Design review of the part built by this model. Coordinates are the model's own, in mm. Face numbers are marked on the shaded views. A direction names the side the tool comes from. Round coordinates to 2 decimals unless told otherwise and drop trailing zeros. Loops run counter-clockwise (first coordinate to the right, second up) from the corner with the lowest first, then second, coordinate; pieces in that order, holes last. Notation, with made-up numbers: (56.5, 40) - (73.5, 40) arc R21 cw to (73.5, 54) - close; hole circle Ø5 at (-25, 74). An arc over 180 degrees is marked (long way). Use one line per item in the form item = value. Start each with the question number.
(1) We need section C-C, the plane z = 3. Write out the cut boundary in (x, y).
(2) We need section D-D, the plane z = 16. Write out the cut boundary in (x, y).
(3) The part is to be moulded in two halves that separate along X. For the marked faces 6, 7, 8 and 9, say which applies: released by +X, released by -X, zero draft, split by the parting line, or undercut.
(4) We need section A-A, the plane y = -40. Write out the cut boundary in (x, z), then the cut area to 3 significant figures.
(5) For pin 1 (5 mm diameter, centred on x = -23.5, y = -33, fed in from -Z); pin 2 (4 mm diameter, centred on x = 20.5, y = -42.5, fed in from +Z); pin 3 (9.5 mm diameter, centred on x = -24, y = -44, fed in from +Z), all flat-tipped, find the tip position at first contact; note any pin that passes through.
(6) Machinability: for the marked faces 1, 2, 3, 4 and 5, which of the approach directions +Z, -Z, +X, -X, +Y, -Y give a long, thin tool a straight path to every point of the face, cutting with its end or side? Answer none if there is none.
(7) Wall thickness on probe 1 along Y at (x, z) = (1.5, 14); probe 2 along Y at (x, z) = (4, 12.25); probe 3 along Z at (x, y) = (-19, -17.5): over which ranges is each line inside the solid? List them lowest first. Write a range as [from, to].
(8) We need section B-B, the plane x = -8.5. Write out the cut boundary in (y, z), then the cut area to 3 significant figures.
from build123d import *

# Parameters (mm, degrees)
F0_W      = 100
F0_H      = 60
F1_DEPTH  = 31
F3_DEPTH  = 60.001
F4_W      = 30.1
F4_H      = 44.45
F5_DEPTH  = 26.0514508643
F6_W      = 3.4385170311
F6_H      = 44.45
F7_DEPTH  = 8.2
F8_DEPTH  = 2.2
F9_DEPTH  = 22
F10_W     = 3.7688823059
F10_H     = 44.2940850452
F11_DEPTH = 3.6
F12_W     = 35.5
F12_H     = 4.5
F13_DEPTH = 3.7
F14_DEPTH = 0.8
F15_W     = 12
F15_H     = 44.45
F17_DEPTH = 0.7
F18_W     = 10
F18_H     = 44.45
F19_DEPTH = 0.7
F21_DEPTH = 70.6


with BuildPart() as f1:
    # F0 (on Top) → F1 (new body)
    with BuildSketch(Plane.XY):
        with Locations((0.4987093992, -30)):
            Rectangle(F0_W, F0_H)
    extrude(amount=F1_DEPTH)

    # F2 (on face) → F3 (cut, through all)
    with BuildSketch(Plane.XZ.offset(60)):
        Polygon((-49.5012906008, 26.9820707818), (50.4987093992, 0), (50.4987093992, 31), (-49.5012906008, 31), align=None)
    extrude(amount=-F3_DEPTH, mode=Mode.SUBTRACT)

    # F4 (on face) → F5 (cut, through all)
    with BuildSketch(Plane(origin=(3.4269736671, 0, 12.7009290534), x_dir=(0.9654726309, 0, -0.2605045086), z_dir=(0.2605045086, 0, 0.9654726309))):
        with Locations((-1.0446142405, -30.225)):
            Rectangle(F4_W, F4_H)
    extrude(amount=-F5_DEPTH, mode=Mode.SUBTRACT)

    # F6 (on face) → F7 (cut)
    with BuildSketch(Plane(origin=(3.4269736671, 0, 12.7009290534), x_dir=(0.9654726309, 0, -0.2605045086), z_dir=(0.2605045086, 0, 0.9654726309))):
        with Locations((-17.8138727561, -30.225)):
            Rectangle(F6_W, F6_H)
    extrude(amount=-F7_DEPTH, mode=Mode.SUBTRACT)

    # F8 (add): a face of the model
    f8_faces = [f1.faces().sort_by_distance(p)[0] for p in [
        (15.7275193268, -30.225, 4.5262314589),
    ]]
    extrude(f8_faces, amount=F8_DEPTH)

    # F9 (cut): a face of the model
    f9_faces = [f1.faces().sort_by_distance(p)[0] for p in [
        (-49.5012906008, -30, 13.4910353909),
    ]]
    extrude(f9_faces, amount=-F9_DEPTH, mode=Mode.SUBTRACT)

    # F10 (on face) → F11 (join)
    with BuildSketch(Plane(origin=(3.4269736671, 0, 12.7009290534), x_dir=(0.9654726309, 0, -0.2605045086), z_dir=(0.2605045086, 0, 0.9654726309))):
        with Locations((13.6898269124, -30.3029574774)):
            Rectangle(F10_W, F10_H)
    extrude(amount=F11_DEPTH)

    # F12 (on face) → F13 (join)
    with BuildSketch(Plane(origin=(3.4269736671, 0, 12.7009290534), x_dir=(0.9654726309, 0, -0.2605045086), z_dir=(0.2605045086, 0, 0.9654726309))):
        with Locations((-1.7831312716, -2.25)):
            Rectangle(F12_W, F12_H)
        with Locations((-1.7831312716, -57.75)):
            Rectangle(F12_W, F12_H)
    extrude(amount=F13_DEPTH)

    # F14 (add): a face of the model
    f14_faces = [f1.faces().sort_by_distance(p)[0] for p in [
        (17.5819431037, -30.3029574774, 12.6103688914),
    ]]
    extrude(f14_faces, amount=F14_DEPTH)

    # F15 (on face) → F17 (cut)
    with BuildSketch(Plane(origin=(0, 0, 0), x_dir=(1, 0, 0), z_dir=(0, 0, -1))):
        with Locations((26.5654576292, 30.3591284901)):
            Rectangle(F15_W, F15_H)
    extrude(amount=-F17_DEPTH, mode=Mode.SUBTRACT)

    # F18 (on face) → F19 (cut)
    with BuildSketch(Plane(origin=(0, 0, 0), x_dir=(1, 0, 0), z_dir=(0, 0, -1))):
        with Locations((-21.6701921171, 30.225)):
            Rectangle(F18_W, F18_H)
    extrude(amount=-F19_DEPTH, mode=Mode.SUBTRACT)

    # F20 (on face) → F21 (cut)
    with BuildSketch(Plane.XZ.offset(60)):
        Polygon((-27.5012906008, 17.7893978176), (-15.431729971, 17.7893978176), (-27.5012906008, 21.0460152098), align=None)
    extrude(amount=-F21_DEPTH, mode=Mode.SUBTRACT)


solid = f1.part
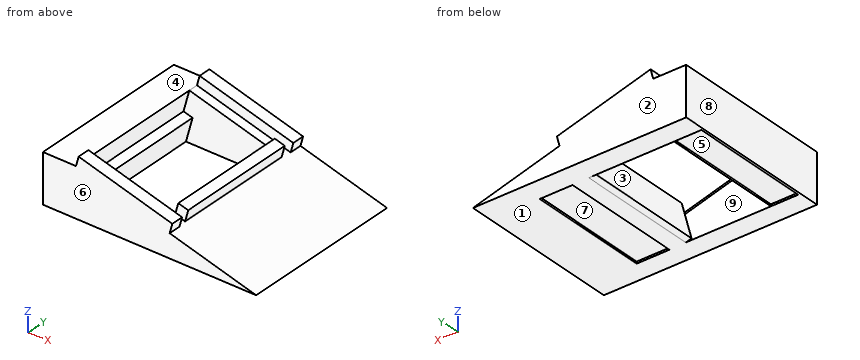
Data:
q1.outline = (-27.5, -60) - (39.38, -60) - (39.38, 0) - (-27.5, 0) - close; hole (-15.86, -52.45) - (13.04, -52.45) - (13.04, -8) - (-15.86, -8) - close
q2.outline = (-27.5, -60) - (5.4, -60) - (5.4, -55.5) - (-8.8, -55.5) - (-8.8, -52.45) - (-15.91, -52.45) - (-15.91, -8) - (-8.8, -8) - (-8.8, -4.5) - (5.4, -4.5) - (5.4, 0) - (-27.5, 0) - close
q3.face_6 = zero draft
q3.face_7 = undercut
q3.face_8 = released by -X
q3.face_9 = undercut
q4.outline = (-27.5, 0) - (-26.67, 0) - (-26.67, 0.7) - (-16.67, 0.7) - (-16.67, 0) - (-14.25, 8.98) - (-17.57, 9.87) - (-15.43, 17.79) - (-27.5, 17.79) - close; (12.38, 0.57) - (14.51, 0) - (20.57, 0) - (20.57, 0.7) - (32.57, 0.7) - (32.57, 0) - (50.5, 0) - (18.46, 8.64) - (19.61, 12.89) - (15.97, 13.87) - close
q4.area = 390 mm^2
q5.pin_1 = 0.7
q5.pin_2 = 13.19
q5.pin_3 = 17.79
q6.face_1 = -Z, +X, -X, +Y, -Y
q6.face_2 = +Z, -Z, +X, -X, +Y
q6.face_3 = +Z
q6.face_4 = +Z, -X, +Y, -Y
q6.face_5 = -Z
q7.probe_1 = [-60, -55.5], [-4.5, 0]
q7.probe_2 = [-60, -52.45], [-8, 0]
q7.probe_3 = [0.7, 17.79]
q8.outline = (-60, 0) - (-52.45, 0) - (-52.45, 15.92) - (-55.5, 15.92) - (-55.5, 19.75) - (-60, 19.75) - close; (-8, 0) - (0, 0) - (0, 19.75) - (-4.5, 19.75) - (-4.5, 15.92) - (-8, 15.92) - close
q8.area = 282 mm^2
